Part print with two shaded views. Sizes in mm from the minimum x, y, z corner. Round coordinates to 2 decimals unless told otherwise and drop trailing zeros. Loops run counter-clockwise (first coordinate to the right, second up) from the corner with the lowest first, then second, coordinate; pieces in that order, holes last. Notation, with made-up numbers: (48, 51.5) -> (56, 51.5) arc R28 ccw to (56, 88.5) -> close; hole circle Ø8 at (74.5, 54). An arc over 180 degrees is marked (long way). Put each result on its own line as item: value. Start each with the question number.
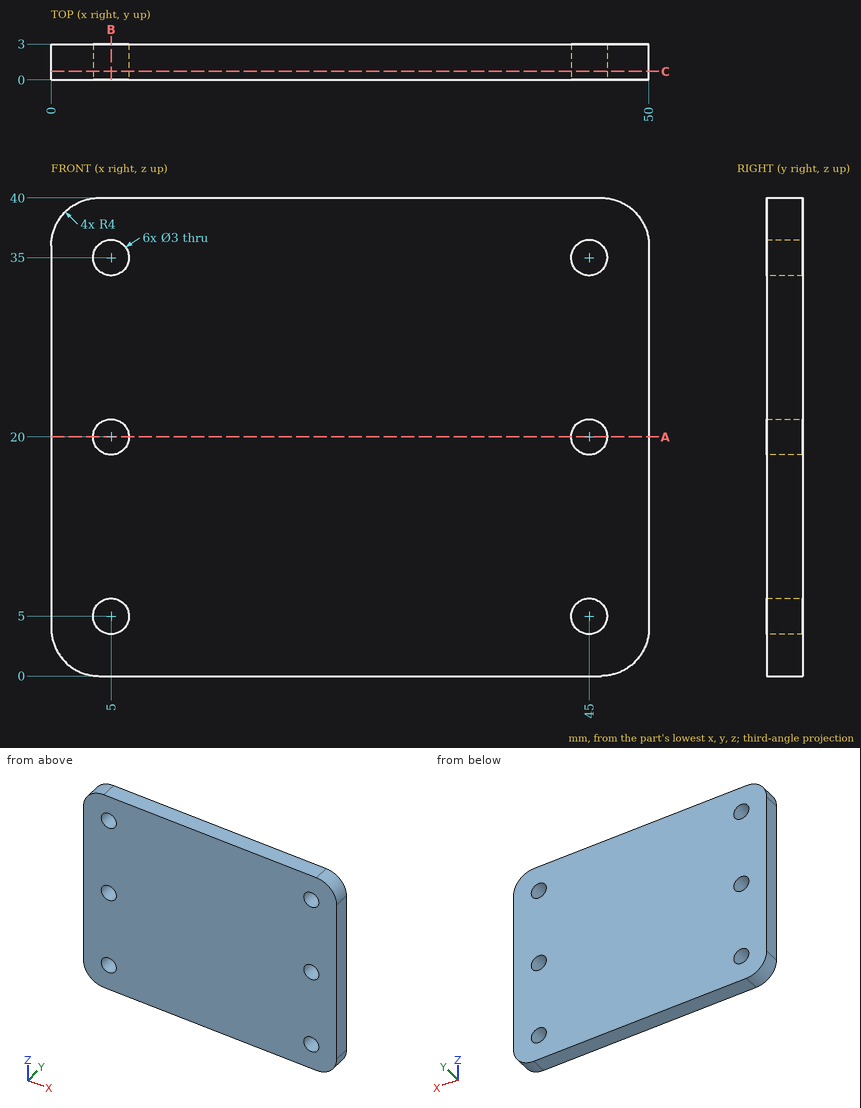
Item 1: Wall check: line 1 (X direction, y = 0.9, z = 5); line 2 (Z direction, x = 6, y = 2.15); line 3 (X direction, y = 0.8, z = 34). Give the ranges that are in metal, low to high. Write a range as from..to.
Item 2: Cut at C-C on y = 0.7. Write the cut outline in (x, z), then the cut area to 3 significant figures.
Item 3: Cut at A-A on z = 20. Write the cut outline in (x, y).
Item 4: Drop a flat-ended pin along its axis: pin 1 (4 mm diameter, centred on x = 5, z = 35, fed in from +Y). Give the stop position or say it passes through.
Item 5: Cut at B-B on x = 5. Write the cut outline in (y, z), then the cut area to 3 significant figures.
Ans:
1. line 1: x = 0..3.5, 6.5..43.5, 46.5..50
1. line 2: z = 0..3.88, 6.12..18.88, 21.12..33.88, 36.12..40
1. line 3: x = 0..3.88, 6.12..43.88, 46.12..50
2. outline: (0, 4) arc R4 ccw to (4, 0) -> (46, 0) arc R4 ccw to (50, 4) -> (50, 36) arc R4 ccw to (46, 40) -> (4, 40) arc R4 ccw to (0, 36) -> close; hole circle Ø3 at (5, 5); hole circle Ø3 at (5, 20); hole circle Ø3 at (5, 35); hole circle Ø3 at (45, 5); hole circle Ø3 at (45, 20); hole circle Ø3 at (45, 35)
2. area: 1,940 mm2
3. outline: (0, 0) -> (3.5, 0) -> (3.5, 3) -> (0, 3) -> close; (6.5, 0) -> (43.5, 0) -> (43.5, 3) -> (6.5, 3) -> close; (46.5, 0) -> (50, 0) -> (50, 3) -> (46.5, 3) -> close
4. pin 1: stops at y = 3
5. outline: (0, 0) -> (3, 0) -> (3, 3.5) -> (0, 3.5) -> close; (0, 6.5) -> (3, 6.5) -> (3, 18.5) -> (0, 18.5) -> close; (0, 21.5) -> (3, 21.5) -> (3, 33.5) -> (0, 33.5) -> close; (0, 36.5) -> (3, 36.5) -> (3, 40) -> (0, 40) -> close
5. area: 93.0 mm2
